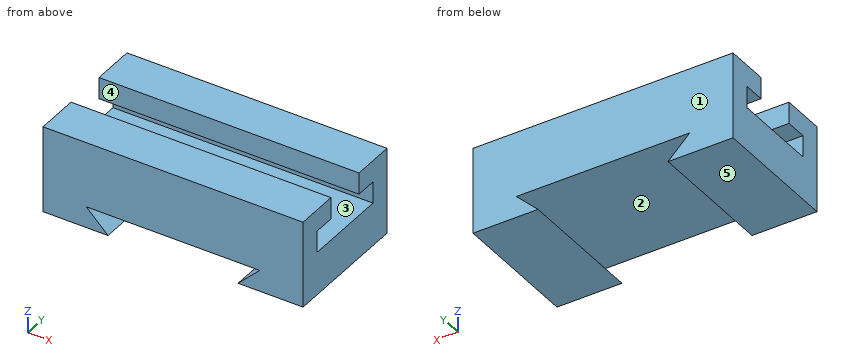
```python
from build123d import *

# Parameters (mm, degrees)
F1_DEPTH = 152.4
F4_DEPTH = 76.2


with BuildPart() as f1:
    # F0 (on Right) → F1 (new body)
    with BuildSketch(Plane.YZ):
        Polygon((-41.44403, 50.8), (-41.44403, 0), (34.75597, 0), (34.75597, 50.8), (9.35597, 50.8), (9.35597, 38.1), (22.05597, 38.1), (22.05597, 25.4), (-28.74403, 25.4), (-28.74403, 38.1), (-16.04403, 38.1), (-16.04403, 50.8), align=None)
    extrude(amount=F1_DEPTH)

    # F3 (on face) → F4 (cut, through all)
    with BuildSketch(Plane(origin=(0, 34.75597, 0), x_dir=(-1, 0, 0), z_dir=(0, 1, 0))):
        Polygon((-127, 12.443408), (-114.3, 0), (-38.1, 0), (-25.4, 12.443408), align=None)
    extrude(amount=-F4_DEPTH, mode=Mode.SUBTRACT)


solid = f1.part
```
Input: part model. Units: mm. Frame: model coordinates. Face numbers are marked on the shaded views. A direction names the side the tool comes from. Give positions to 0.01 mm unless a question says otherwise; leave off trailing zeros. Order: outer loops, then holes, each group sorted by start corner. A loop starts at its lowest first (then second) coordinate and runs counter-clockwise, first axis right, second up. Notation, with made-up numbers: (16, -17) - (22, -17) arc R27 cw to (22, 6) - close; hole circle Ø11 at (47, -12). An arc over 180 degrees is marked (long way). Put each result on its own line as item: value.
Item 1: Contact query for flat-ended pins moving along their axis: pin 1 (15 mm diameter, centred on x = 52.5, y = -3.5, fed in from +Z); pin 2 (4 mm diameter, centred on x = 98.5, y = 16, fed in from -Z). Output: stop coordinate, or through.
Found:
pin 1: stops at z = 25.4
pin 2: stops at z = 12.44
Item 2: Section query D-D, the plane x = 31.5. Return loops of the section in (y, z), then the cut area to 3 significant figures.
Found:
outline: (-41.44, 0) - (34.76, 0) - (34.76, 6.47) - (-41.44, 6.47) - close; (-41.44, 12.44) - (34.76, 12.44) - (34.76, 50.8) - (9.36, 50.8) - (9.36, 38.1) - (22.06, 38.1) - (22.06, 25.4) - (-28.74, 25.4) - (-28.74, 38.1) - (-16.04, 38.1) - (-16.04, 50.8) - (-41.44, 50.8) - close
area: 2,450 mm^2
Item 3: Section query C-C, the plane y = -20. Return loops of the section in (x, z), then the cut area to 3 significant figures.
Found:
outline: (0, 0) - (38.1, 0) - (25.4, 12.44) - (127, 12.44) - (114.3, 0) - (152.4, 0) - (152.4, 25.4) - (0, 25.4) - close; (0, 38.1) - (152.4, 38.1) - (152.4, 50.8) - (0, 50.8) - close
area: 4,700 mm^2
Item 4: Section query A-A, the plane z = 44. Return loops of the section in (x, y), then the cut area to 3 significant figures.
Found:
outline: (0, -41.44) - (152.4, -41.44) - (152.4, -16.04) - (0, -16.04) - close; (0, 9.36) - (152.4, 9.36) - (152.4, 34.76) - (0, 34.76) - close
area: 7,740 mm^2
Item 5: Section query B-B, the plane x = 10.5. Return loops of the section in (y, z), then the cut area to 3 significant figures.
Found:
outline: (-41.44, 0) - (34.76, 0) - (34.76, 50.8) - (9.36, 50.8) - (9.36, 38.1) - (22.06, 38.1) - (22.06, 25.4) - (-28.74, 25.4) - (-28.74, 38.1) - (-16.04, 38.1) - (-16.04, 50.8) - (-41.44, 50.8) - close
area: 2,900 mm^2
Item 6: Draft query along Y for the marked faces 1, 2 and 3. Return one class per face: +Y half, -Y half, draft (parallel to the pull), parting line (faces both ways), or undercut.
Found:
face 1: +Y half
face 2: draft
face 3: undercut
Item 7: Ray query, L1, parallel to Y at x = 85, z = 47.5; L2, parallel to Y at x = 24, z = 38; L3, parallel to Z at x = 26, y = 13. Return the intervals inside material, ascending. Write a range as from..to.
Found:
L1: y = -41.44..-16.04, 9.36..34.76
L2: y = -41.44..-28.74, 22.06..34.76
L3: z = 0..11.86, 12.44..25.4, 38.1..50.8
Item 8: Access query for the marked faces 4 and 5. Directions: +Z, -Z, +X, -X, +Y, -Y. A direction counts if a zero-diameter tool reaches every point of the face in a straight line with its end or side. Return the directions, or none.
Found:
face 4: +Z, +X, -X
face 5: -Z, +X, -X, +Y, -Y
